from build123d import *

# Parameters (mm, degrees)
BOSS_EXTRUDE1_DEPTH = 2.7


with BuildPart() as part:
    # Sketch1 → Boss-Extrude1 (new body)
    with BuildSketch(Plane.XY):
        with BuildLine():
            Line((-103.5, 126.6), (103.5, 126.6))
            ThreePointArc((103.5, 126.6), (110.571067812, 123.671067812), (113.5, 116.6))
            Line((113.5, 116.6), (113.5, -116.6))
            ThreePointArc((113.5, -116.6), (110.571067812, -123.671067812), (103.5, -126.6))
            Line((103.5, -126.6), (33.149945785, -126.6))
            Line((33.149945785, -126.6), (33.149945785, -86.203548192))
            ThreePointArc((33.149945785, -86.203548192), (-2.1875, -50.866102407), (-37.524945785, -86.203548192))
            Line((-37.524945785, -86.203548192), (-37.524945785, -126.6))
            Line((-37.524945785, -126.6), (-103.5, -126.6))
            ThreePointArc((-103.5, -126.6), (-110.571067812, -123.671067812), (-113.5, -116.6))
            Line((-113.5, -116.6), (-113.5, 116.6))
            ThreePointArc((-113.5, 116.6), (-110.571067812, 123.671067812), (-103.5, 126.6))
        make_face()
    extrude(amount=BOSS_EXTRUDE1_DEPTH)


solid = part.part
Geometry: final body of the model. Coordinates: model frame, mm. Coordinates: 2 decimals unless noted, no trailing zeros. Order: outer loops, then holes, each group sorted by start corner. A loop starts at its lowest first (then second) coordinate and runs counter-clockwise, first axis right, second up.
1) Section C-C (x = 27.5). Return loops of the section in (y, z).
Result sheet:
outline: (-67.04, 0) - (126.6, 0) - (126.6, 2.7) - (-67.04, 2.7) - close
2) Ray query, probe 1 along X at (y, z) = (-70.5, 1.45); probe 2 along X at (y, z) = (-71, 0.2); probe 3 along Y at (x, z) = (-104, 1.9). Return the intervals inside material, ascending.
Result sheet:
probe 1: x = -113.5 to -33.84, 29.47 to 113.5
probe 2: x = -113.5 to -34.09, 29.71 to 113.5
probe 3: y = -126.59 to 126.59
3) Draft query along X for faces 1 (the cylindrical face through (-1.41, -50.875, 1.331)), 2 (the flat face through (2, 2, 2.7)), 3 (the cylindrical face through (110.65, -123.59, 1.33)), 4 (the cylindrical face through (-110.49, -123.75, 1.33)). Return one class per face: released by +X, released by -X, zero draft, split by the parting line, or undercut.
Result sheet:
face 1: undercut
face 2: zero draft
face 3: released by +X
face 4: released by -X
4) Section A-A (z = 0.5). Return loops of the section in (x, y), then the cut area to 3 significant figures.
Result sheet:
outline: (-113.5, -116.6) arc R10 ccw to (-103.5, -126.6) - (-37.52, -126.6) - (-37.52, -86.2) arc R35.34 cw to (33.15, -86.2) - (33.15, -126.6) - (103.5, -126.6) arc R10 ccw to (113.5, -116.6) - (113.5, 116.6) arc R10 ccw to (103.5, 126.6) - (-103.5, 126.6) arc R10 ccw to (-113.5, 116.6) - close
area: 52,600 mm2
5) Section B-B (x = -28.5). Return loops of the section in (y, z), then the cut area to 3 significant figures.
Result sheet:
outline: (-62.62, 0) - (126.6, 0) - (126.6, 2.7) - (-62.62, 2.7) - close
area: 511 mm2
